Geometry: final body of the model. Coordinates: model frame, mm. Round coordinates to 2 decimals unless told otherwise and drop trailing zeros. Loops run counter-clockwise (first coordinate to the right, second up) from the corner with the lowest first, then second, coordinate; pieces in that order, holes last. Notation, with made-up numbers: M 57.25,49 L 64.25,49 A19 cw 64.25,62 Z; hole C -39.75,-1.75 d2. An arc over 180 degrees is marked long. Write each question's results on one line, items separated by ' | '.
```python
from build123d import *

# Parameters (mm, degrees)
F1_W     = 400
F1_H     = 524
F1_R     = 2.5
F1_R_2   = 6
F1_H_2   = 12
F1_H_3   = 60
F2_DEPTH = 12


with BuildPart() as f2:
    # F1 (on Front) → F2 (new body)
    with BuildSketch(Plane.XZ):
        with Locations((0, 112)):
            Rectangle(F1_W, F1_H)
        with Locations((-175, 293)):
            Circle(F1_R, mode=Mode.SUBTRACT)
        with Locations((-175, 312)):
            Circle(F1_R_2, mode=Mode.SUBTRACT)
        with Locations((-175, 331)):
            Circle(F1_R, mode=Mode.SUBTRACT)
        with BuildLine():
            Line((-150, 278), (90, 278))
            ThreePointArc((90, 278), (104.1421356237, 272.1421356237), (110, 258))
            Line((110, 258), (110, 162))
            ThreePointArc((110, 162), (115.8578643763, 147.8578643763), (130, 142))
            Line((130, 142), (150, 142))
            ThreePointArc((150, 142), (164.1421356237, 136.1421356237), (170, 122))
            Line((170, 122), (170, -120))
            ThreePointArc((170, -120), (164.1421356237, -134.1421356237), (150, -140))
            Line((150, -140), (-150, -140))
            ThreePointArc((-150, -140), (-164.1421356237, -134.1421356237), (-170, -120))
            Line((-170, -120), (-170, 258))
            ThreePointArc((-170, 258), (-164.1421356237, 272.1421356237), (-150, 278))
        make_face(mode=Mode.SUBTRACT)
        with Locations((175, 293)):
            Circle(F1_R, mode=Mode.SUBTRACT)
        with Locations((175, 312)):
            Circle(F1_R_2, mode=Mode.SUBTRACT)
        with Locations((175, 331)):
            Circle(F1_R, mode=Mode.SUBTRACT)
        with Locations((0, -156)):
            Rectangle(F1_W, F1_H_2)
        with Locations((0, -192)):
            Rectangle(F1_W, F1_H_3)
        Polygon((200, -234), (200, -222), (-200, -222), (-200, -234), (-150, -234), (150, -234), align=None)
        with BuildLine():
            Line((200, -260), (200, -234))
            Line((200, -234), (150, -234))
            ThreePointArc((150, -234), (164.1421356237, -239.8578643763), (170, -254))
            Line((170, -254), (170, -260))
            Line((170, -260), (200, -260))
        make_face()
        with BuildLine():
            Line((-150, -234), (-200, -234))
            Line((-200, -234), (-200, -260))
            Line((-200, -260), (-170, -260))
            Line((-170, -260), (-170, -254))
            ThreePointArc((-170, -254), (-164.1421356237, -239.8578643763), (-150, -234))
        make_face()
    extrude(amount=F2_DEPTH)


solid = f2.part
```
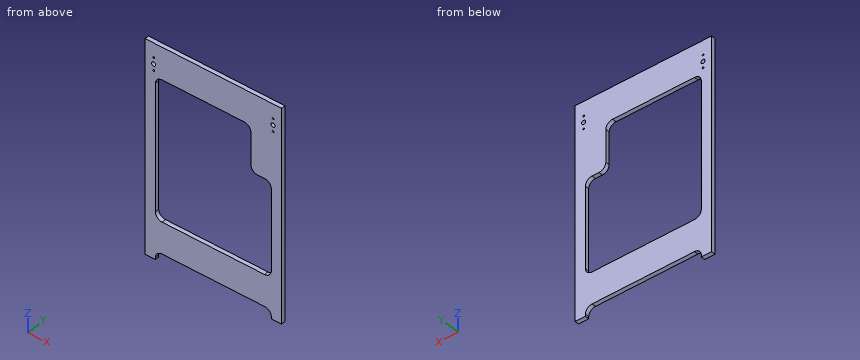
1. Ray query, probe 1 along X at (y, z) = (-4.5, 293); probe 2 along Z at (x, y) = (175, -4); probe 3 along X at (y, z) = (-2.25, 312). Return the intervals inside material, ascending.
Answer key:
probe 1: x = -200 to -177.5, -172.5 to 172.5, 177.5 to 200 | probe 2: z = -260 to 290.5, 295.5 to 306, 318 to 328.5, 333.5 to 374 | probe 3: x = -200 to -181, -169 to 169, 181 to 200
2. Section D-D (x = 23). Output: boundary loops of the cut face in (y, z).
Answer key:
outline: M -12,-234 L 0,-234 L 0,-140 L -12,-140 Z; M -12,278 L 0,278 L 0,374 L -12,374 Z
3. Section B-B (y = -2.5). Output: boundary loops of the cut face in (x, z).
Answer key:
outline: M -200,-260 L -170,-260 L -170,-254 A20 cw -150,-234 L 150,-234 A20 cw 170,-254 L 170,-260 L 200,-260 L 200,374 L -200,374 Z; hole C -175,312 d12; hole C -175,293 d5; hole C -175,331 d5; hole M -170,-120 A20 ccw -150,-140 L 150,-140 A20 ccw 170,-120 L 170,122 A20 ccw 150,142 L 130,142 A20 cw 110,162 L 110,258 A20 ccw 90,278 L -150,278 A20 ccw -170,258 Z; hole C 175,312 d12; hole C 175,293 d5; hole C 175,331 d5
4. Section A-A (z = 312). Output: boundary loops of the cut face in (x, y).
Answer key:
outline: M -200,-12 L -181,-12 L -181,0 L -200,0 Z; M -169,-12 L 169,-12 L 169,0 L -169,0 Z; M 181,-12 L 200,-12 L 200,0 L 181,0 Z
5. Pin query (flat end, axial travel): P1, Ø6, axis at x = 175, z = 293, coming from the +Y side; P2, Ø9.5, axis at x = 175, z = 312, coming from the -Y side; P3, Ø5, axis at x = 150.5, y = -5.5, coming from the -Z side; P4, Ø3, axis at x = -154, y = -10.5, coming from the -Z side. Return the tip coordinate at first contact, or that it passes through.
Answer key:
P1: stops at y = 0 | P2: passes through | P3: stops at z = -234.23 | P4: stops at z = -234.77
6. Section C-C (z = 29.5). Output: boundary loops of the cut face in (x, y), then the cut area to 3 significant figures.
Answer key:
outline: M -200,-12 L -170,-12 L -170,0 L -200,0 Z; M 170,-12 L 200,-12 L 200,0 L 170,0 Z | area: 720 mm²
